Autodesk Inventor part; units mm, degrees
ref_plane "YZ Plane" through (0, 0, 0) normal (1, 0, 0) x (0, 1, 0)
ref_plane "XZ Plane" through (0, 0, 0) normal (0, 1, 0) x (-1, 0, 0)
ref_plane "XY Plane" through (0, 0, 0) normal (0, 0, 1) x (1, 0, 0)
sketch "Boceto1" plane through (0, 0, 0) normal (0, 1, 0) x (-1, 0, 0)
  line L0 (50, 469.5) -> (-50, 469.5)
  line L1 (-50, 469.5) -> (-50, -469.5)
  line L2 (-50, -469.5) -> (50, -469.5)
  line L3 (50, -469.5) -> (50, 469.5)
  line L4 (0, 469.5) -> (0, 0) construction
  line L5 (0, 0) -> (-50, 0) construction
  dimension "d0" = 100
  dimension "d1" = 939
extrude "Extrusión1" add sketch "Boceto1" along normal blind 19
sketch "Boceto2" plane through (0, 19, 0) normal (0, 1, 0) x (1, 0, 0)
  line L0 (-50, -469.5) -> (50, -469.5)
  line L1 (-10, -469.5) -> (10, -469.5)
  line L2 (10, -469.5) -> (10, 469.5)
  line L3 (10, 469.5) -> (-10, 469.5)
  line L4 (-10, 469.5) -> (-10, -469.5)
  line L5 (50, 469.5) -> (-50, 469.5)
  point P0 (0, 0)
  point P1 (0, -469.5)
  dimension "d4" = 20
extrude "Extrusión2" add sketch "Boceto2" along normal blind 48
sketch "Boceto3" plane through (0, 0, 0) normal (0, -1, 0) x (1, 0, 0)
  line L0 (50, 469.5) -> (50, -469.5)
  line L1 (50, -464) -> (-50, -464) construction
  line L2 (-50, -469.5) -> (-50, 469.5)
  circle A0 centre (36.5, -464) radius 1.5
  circle A1 centre (13.5, -464) radius 1.5
  line L3 (50, -469.5) -> (-50, -469.5)
  line L4 (50, -464) -> (0, -464) construction
  line L5 (25, -464) -> (25, -433.7226) construction
  line L6 (0, -464) -> (0, -462.9029) construction
  circle A2 centre (-36.5, -464) radius 1.5
  circle A3 centre (-13.5, -464) radius 1.5
  point P0 (0, 0)
  dimension "d7" = 3
  dimension "d8" = 5.5
  dimension "d9" = 23
extrude "Extrusión3" cut sketch "Boceto3" against normal through all
ref_plane "Plano de trabajo1" through (50, 0, 0) normal (0, 0, -1) x (-1, 0, 0)
mirror "Simetría1" about plane through (50, 0, 0) normal (0, 0, -1) of "Extrusión3"
properties part number "Madera" material "Madera (abedul)"
Geometry check sheet. Reference: the model listing, model coordinates, mm. A direction names the side the tool comes from. Give positions to 0.01 mm unless a question says otherwise; leave off trailing zeros. Loops run counter-clockwise (first coordinate to the right, second up) from the corner with the lowest first, then second, coordinate; pieces in that order, holes last. Notation, with made-up numbers: M 71.25,36.5 L 110.25,36.5 A9 ccw 110.25,42.5 Z; hole C 75.25,-25 d9. An arc over 180 degrees is marked long. Answer as CSV lines item,"result".
Item 1: Access from +Z, -Z, +X, -X, +Y, -Y to the whole of each face (thin tool, end or side, straight path). Record for faces 1 (the flat face through (-10, 43, -7)), 2 (the flat face through (50, 9, 7)), 3 (the flat face through (10, 43, 7)).
Values:
face 1,"+Z, -Z, -X, +Y"
face 2,"+Z, -Z, +X, +Y, -Y"
face 3,"+Z, -Z, +X, +Y"
Item 2: Depth check by flat-ended pin: P1, Ø12, axis at y = 49, z = -119.5, coming from the +X side; P2, Ø4, axis at x = 17.5, z = -340, coming from the +Y side; P3, Ø5, axis at y = 55.5, z = 301.5, coming from the -X side. Enter the tip coordinate at first touch or a pass-through.
Values:
P1,"stops at x = 10"
P2,"stops at y = 19"
P3,"stops at x = -10"
Item 3: Material ranges on line 1 (X direction, y = 14, z = 464); line 2 (Z direction, x = 36, y = 15); line 3 (Z direction, x = 36.5, y = 5.5), recorded low to high.
Values:
line 1,"x = -50 to -38, -35 to -15, -12 to 12, 15 to 35, 38 to 50"
line 2,"z = -469.5 to -465.41, -462.59 to 462.59, 465.41 to 469.5"
line 3,"z = -469.5 to -465.5, -462.5 to 462.5, 465.5 to 469.5"
Item 4: Cross-section at B-B on y = 53.5. Record the cut outline in (x, z).
Values:
outline,"M -10,-469.5 L 10,-469.5 L 10,469.5 L -10,469.5 Z"
Item 5: Cross-section at A-A on z = -83.5. Record the cut outline in (x, y).
Values:
outline,"M -50,0 L 50,0 L 50,19 L 10,19 L 10,67 L -10,67 L -10,19 L -50,19 Z"
